Source: CAD feature listing. Evaluate the final solid. Frame: model axes, mm. A direction names the side the tool comes from. Round coordinates to 2 decimals unless told otherwise and drop trailing zeros. Order: outer loops, then holes, each group sorted by start corner. A loop starts at its lowest first (then second) coordinate and runs counter-clockwise, first axis right, second up. Notation, with made-up numbers: (6, -15.75) -> (65, -15.75) arc R16 cw to (65, 15.25) -> close; hole circle Ø8 at (-10.5, 57.5). An arc over 180 degrees is marked (long way). Answer as CSV lines item,"result".
from build123d import *

# Parameters (mm, degrees)
F0_W      = 38.1
F0_H      = 55.88
F1_DEPTH  = 5.08
F2_W      = 38.1
F2_H      = 2.54
F3_DEPTH  = 38.1
F5_W      = 3.81
F5_H      = 25.4
F6_DEPTH  = 38.1
F7_W      = 3.81
F7_H      = 25.4
F8_DEPTH  = 38.1
F10_DEPTH = 127
F11_DEPTH = 25.4
F12_DEPTH = 25.4
F14_DEPTH = 25.4
F16_DEPTH = 25.4


with BuildPart() as f1:
    # F0 (on Top) → F1 (new body)
    with BuildSketch(Plane.XY):
        with Locations((19.05, 27.94)):
            Rectangle(F0_W, F0_H)
    extrude(amount=F1_DEPTH)

    # F2 (on face) → F3 (join)
    with BuildSketch(Plane.XY.offset(5.08)):
        with Locations((19.05, 29.21)):
            Rectangle(F2_W, F2_H)
        with Locations((19.05, 26.67)):
            Rectangle(F2_W, F2_H)
    extrude(amount=F3_DEPTH)

    # F5 (on face) → F6 (join)
    with BuildSketch(Plane.XY.offset(5.08)):
        with Locations((1.905, 12.7)):
            Rectangle(F5_W, F5_H)
        with Locations((36.195, 12.7)):
            Rectangle(F5_W, F5_H)
    extrude(amount=F6_DEPTH)

    # F7 (on face) → F8 (join)
    with BuildSketch(Plane.XY.offset(5.08)):
        with Locations((36.195, 43.18)):
            Rectangle(F7_W, F7_H)
        with Locations((1.905, 43.18)):
            Rectangle(F7_W, F7_H)
    extrude(amount=F8_DEPTH)

    # F9 (on face) → F10 (cut)
    with BuildSketch(Plane(origin=(0, 0, 0), x_dir=(0, -1, 0), z_dir=(-1, 0, 0))):
        Polygon((-55.88, 43.18), (-55.88, 11.43), (-30.48, 30.48), (-30.48, 43.18), align=None)
        Polygon((0, 43.18), (-25.4, 43.18), (-25.4, 30.48), (0, 11.43), align=None)
    extrude(amount=-F10_DEPTH, mode=Mode.SUBTRACT)

    # F4 (on face) → F11 (cut)
    with BuildSketch(Plane.XZ.offset(-25.4)):
        with BuildLine():
            ThreePointArc((19.05, 15.2908), (17.78, 14.0208), (19.05, 12.7508))
            Line((19.05, 12.7508), (19.05, 15.2908))
        make_face()
        with BuildLine():
            Line((19.05, 15.2908), (19.05, 12.7508))
            ThreePointArc((19.05, 12.7508), (19.9480256121, 13.1227743879), (20.32, 14.0208))
            ThreePointArc((20.32, 14.0208), (19.9480256121, 14.9188256121), (19.05, 15.2908))
        make_face()
        with BuildLine():
            ThreePointArc((29.5402, 24.13), (30.8102, 22.86), (32.0802, 24.13))
            Line((32.0802, 24.13), (29.5402, 24.13))
        make_face()
        with BuildLine():
            Line((29.5402, 24.13), (32.0802, 24.13))
            ThreePointArc((32.0802, 24.13), (30.8102, 25.4), (29.5402, 24.13))
        make_face()
        with BuildLine():
            ThreePointArc((20.32, 34.2392), (19.9480256121, 35.1372256121), (19.05, 35.5092))
            Line((19.05, 35.5092), (19.05, 32.9692))
            ThreePointArc((19.05, 32.9692), (19.9480256121, 33.3411743879), (20.32, 34.2392))
        make_face()
        with BuildLine():
            Line((19.05, 32.9692), (19.05, 35.5092))
            ThreePointArc((19.05, 35.5092), (17.78, 34.2392), (19.05, 32.9692))
        make_face()
        with BuildLine():
            ThreePointArc((8.5598, 24.13), (7.2898, 25.4), (6.0198, 24.13))
            Line((6.0198, 24.13), (8.5598, 24.13))
        make_face()
        with BuildLine():
            Line((8.5598, 24.13), (6.0198, 24.13))
            ThreePointArc((6.0198, 24.13), (7.2898, 22.86), (8.5598, 24.13))
        make_face()
    extrude(amount=-F11_DEPTH, mode=Mode.SUBTRACT)

    # F4 (on face) → F12 (cut)
    with BuildSketch(Plane.XZ.offset(-25.4)):
        with BuildLine():
            Line((19.05, 26.162), (19.05, 30.48))
            ThreePointArc((19.05, 30.48), (14.5598719395, 28.6201280605), (12.7, 24.13))
            Line((12.7, 24.13), (17.018, 24.13))
            ThreePointArc((17.018, 24.13), (17.6131590206, 25.5668409794), (19.05, 26.162))
        make_face()
        with BuildLine():
            ThreePointArc((25.4, 24.13), (23.5401280605, 28.6201280605), (19.05, 30.48))
            Line((19.05, 30.48), (19.05, 26.162))
            ThreePointArc((19.05, 26.162), (20.4868409794, 25.5668409794), (21.082, 24.13))
            Line((21.082, 24.13), (25.4, 24.13))
        make_face()
        with BuildLine():
            ThreePointArc((21.082, 24.13), (20.4868409794, 25.5668409794), (19.05, 26.162))
            Line((19.05, 26.162), (19.05, 24.13))
            Line((19.05, 24.13), (21.082, 24.13))
        make_face()
        with BuildLine():
            Line((19.05, 24.13), (19.05, 26.162))
            ThreePointArc((19.05, 26.162), (17.6131590206, 25.5668409794), (17.018, 24.13))
            Line((17.018, 24.13), (19.05, 24.13))
        make_face()
        with BuildLine():
            Line((17.018, 24.13), (12.7, 24.13))
            ThreePointArc((12.7, 24.13), (14.5598719395, 19.6398719395), (19.05, 17.78))
            Line((19.05, 17.78), (19.05, 22.098))
            ThreePointArc((19.05, 22.098), (17.6131590206, 22.6931590206), (17.018, 24.13))
        make_face()
        with BuildLine():
            Line((19.05, 24.13), (17.018, 24.13))
            ThreePointArc((17.018, 24.13), (17.6131590206, 22.6931590206), (19.05, 22.098))
            Line((19.05, 22.098), (19.05, 24.13))
        make_face()
        with BuildLine():
            Line((21.082, 24.13), (19.05, 24.13))
            Line((19.05, 24.13), (19.05, 22.098))
            ThreePointArc((19.05, 22.098), (20.4868409794, 22.6931590206), (21.082, 24.13))
        make_face()
        with BuildLine():
            ThreePointArc((19.05, 17.78), (23.5401280605, 19.6398719395), (25.4, 24.13))
            Line((25.4, 24.13), (21.082, 24.13))
            ThreePointArc((21.082, 24.13), (20.4868409794, 22.6931590206), (19.05, 22.098))
            Line((19.05, 22.098), (19.05, 17.78))
        make_face()
    extrude(amount=-F12_DEPTH, mode=Mode.SUBTRACT)

    # F13 (on face) → F14 (cut)
    with BuildSketch(Plane.XY.offset(5.08)):
        with BuildLine():
            ThreePointArc((12.7, 12.7), (10.4267, 14.9733), (8.1534, 12.7))
            Line((8.1534, 12.7), (12.7, 12.7))
        make_face()
        with BuildLine():
            Line((12.7, 12.7), (8.1534, 12.7))
            ThreePointArc((8.1534, 12.7), (10.4267, 10.4267), (12.7, 12.7))
        make_face()
        with BuildLine():
            ThreePointArc((29.9466, 12.7), (27.6733, 14.9733), (25.4, 12.7))
            Line((25.4, 12.7), (29.9466, 12.7))
        make_face()
        with BuildLine():
            Line((29.9466, 12.7), (25.4, 12.7))
            ThreePointArc((25.4, 12.7), (27.6733, 10.4267), (29.9466, 12.7))
        make_face()
    extrude(amount=-F14_DEPTH, mode=Mode.SUBTRACT)

    # F15 (on face) → F16 (cut)
    with BuildSketch(Plane.XY.offset(5.08)):
        with BuildLine():
            ThreePointArc((12.7, 43.18), (10.4267, 45.4533), (8.1534, 43.18))
            Line((8.1534, 43.18), (12.7, 43.18))
        make_face()
        with BuildLine():
            Line((12.7, 43.18), (8.1534, 43.18))
            ThreePointArc((8.1534, 43.18), (10.4267, 40.9067), (12.7, 43.18))
        make_face()
        with BuildLine():
            ThreePointArc((29.9466, 43.18), (27.6733, 45.4533), (25.4, 43.18))
            Line((25.4, 43.18), (29.9466, 43.18))
        make_face()
        with BuildLine():
            Line((29.9466, 43.18), (25.4, 43.18))
            ThreePointArc((25.4, 43.18), (27.6733, 40.9067), (29.9466, 43.18))
        make_face()
    extrude(amount=-F16_DEPTH, mode=Mode.SUBTRACT)


solid = f1.part
1. Mould query, pull axis X, two halves, no side actions, for faces 1 (the flat face through (36.17, 43.36, 20.82)), 2 (the cylindrical face through (9.38, 14.72, 2.58)), 3 (the flat face through (0, 28, 12)). Classes: released by +X, released by -X, zero draft, split by the parting line, or undercut.
Results below:
face 1,"zero draft"
face 2,"undercut"
face 3,"released by -X"
2. Section query A-A on x = 17. Return loops of the section in (y, z).
Results below:
outline,"(0, 0) -> (55.88, 0) -> (55.88, 5.08) -> (30.48, 5.08) -> (30.48, 18.12) -> (25.4, 18.12) -> (25.4, 5.08) -> (0, 5.08) -> close; (25.4, 30.14) -> (30.48, 30.14) -> (30.48, 43.18) -> (25.4, 43.18) -> close"
3. Line query: L1, parallel to X at y = 12.7, z = 3; L2, parallel to Z at x = 31, y = 29; L3, parallel to Y at x = 27.5, z = 3.5. Output: solid intervals per line, ascending. Write a range as [from, to].
Results below:
L1,"[0, 8.15], [12.7, 25.4], [29.95, 38.1]"
L2,"[0, 22.87], [25.39, 43.18]"
L3,"[0, 10.43], [14.97, 40.91], [45.45, 55.88]"
4. Reachability of faces 4 (the flat face through (19, 13, 5.08)), 5 (the flat face through (34.29, 40, 15)), 6 (the flat face through (19, 0, 3)) from +Z, -Z, +X, -X, +Y, -Y: full face, straight path, thin tool, end or side. Return the list, or none.
Results below:
face 4,"+Z, -Y"
face 5,"+Z, +Y"
face 6,"+Z, -Z, +X, -X, -Y"
5. Section query C-C on z = 3. Return loops of the section in (x, y).
Results below:
outline,"(0, 0) -> (38.1, 0) -> (38.1, 55.88) -> (0, 55.88) -> close; hole circle Ø4.55 at (10.43, 12.7); hole circle Ø4.55 at (10.43, 43.18); hole circle Ø4.55 at (27.67, 12.7); hole circle Ø4.55 at (27.67, 43.18)"
6. Section query B-B on y = 6. Return loops of the section in (x, z), and give its area (3 significant figures).
Results below:
outline,"(0, 0) -> (38.1, 0) -> (38.1, 15.93) -> (34.29, 15.93) -> (34.29, 5.08) -> (3.81, 5.08) -> (3.81, 15.93) -> (0, 15.93) -> close"
area,"276 mm2"
7. Pin query (flat end, axial travel): pin 1 (3 mm diameter, centred on x = 30.81, z = 24.13, fed in from +Y); pin 2 (12.5 mm diameter, centred on x = 16.5, y = 12, fed in from +Z); pin 3 (4 mm diameter, centred on x = 4, y = 50, fed in from +Z). Return the tip coordinate at first contact, or that it passes through.
Results below:
pin 1,"y = 30.48"
pin 2,"z = 5.08"
pin 3,"z = 17.33"
8. Section query D-D on z = 20. Return loops of the section in (x, y), and give its area (3 significant figures).
Results below:
outline,"(0, 11.43) -> (3.81, 11.43) -> (3.81, 25.4) -> (14.23, 25.4) -> (14.23, 30.48) -> (3.81, 30.48) -> (3.81, 44.45) -> (0, 44.45) -> close; (23.87, 25.4) -> (34.29, 25.4) -> (34.29, 11.43) -> (38.1, 11.43) -> (38.1, 44.45) -> (34.29, 44.45) -> (34.29, 30.48) -> (23.87, 30.48) -> close"
area,"357 mm2"
